Part model, mm, in its own coordinate system. Face numbers are marked on the shaded views. A direction names the side the tool comes from. Coordinates: 2 decimals unless noted, no trailing zeros. Write each loop counter-clockwise with the first axis right and the second up, starting at its lowest first coordinate (ties: lowest second). Pieces come first, ordered by that corner, then holes. Notation, with made-up numbers: (-3.75, 80) - (46.25, 80) arc R27 ccw to (46.25, 112) - close; hole circle Ø2 at (-3, -13.5). An arc over 180 degrees is marked (long way). Write each question's results on one line, items separated by ' | '.
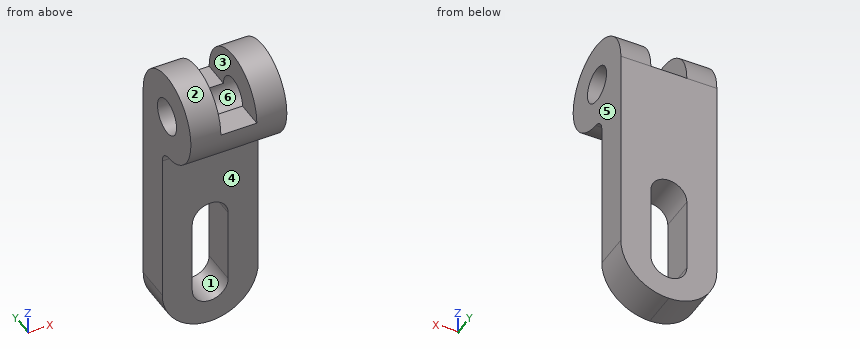
from build123d import *

# Parameters (mm, degrees)
F0_R     = 6
F1_DEPTH = 32
F3_DEPTH = 15.001
F4_W     = 12
F4_H     = 15
F5_DEPTH = 30.001


# Not quite as in the source:
# - a feature names something its author has since deleted; it is built from what else it names


with BuildPart() as f1:
    # F0 (on Right) → F1 (new body)
    with BuildSketch(Plane.YZ):
        with BuildLine():
            Line((15, -86), (15, 0))
            ThreePointArc((15, 0), (-10.3237080242, 10.8821437517), (-0.7894736842, -14.9792099692))
            ThreePointArc((-0.7894736842, -14.9792099692), (1.9019050004, -16.2206771546), (3, -18.973665961))
            Line((3, -18.973665961), (3, -86))
            Line((3, -86), (15, -86))
        make_face()
        Circle(F0_R, mode=Mode.SUBTRACT)
    extrude(amount=-F1_DEPTH)

    # F2 (on Front) → F3 (cut, through all)
    with BuildSketch(Plane.XZ):
        with BuildLine():
            ThreePointArc((-16, -86), (-27.313708499, -81.313708499), (-32, -70))
            Line((-32, -70), (-32, -86))
            Line((-32, -86), (-16, -86))
        make_face()
        with BuildLine():
            ThreePointArc((0, -70), (-4.686291501, -81.313708499), (-16, -86))
            Line((-16, -86), (0, -86))
            Line((0, -86), (0, -70))
        make_face()
        with BuildLine():
            Line((-10, -72.1075447824), (-10, -47.1075447824))
            ThreePointArc((-10, -47.1075447824), (-16, -41.1075447824), (-22, -47.1075447824))
            Line((-22, -47.1075447824), (-22, -72.1075447824))
            ThreePointArc((-22, -72.1075447824), (-16, -78.1075447824), (-10, -72.1075447824))
        make_face()
    extrude(amount=-F3_DEPTH, mode=Mode.SUBTRACT)

    # F4 (on face) → F5 (cut, through all)
    with BuildSketch(Plane(origin=(0, 15, 0), x_dir=(-1, 0, 0), z_dir=(0, 1, 0))):
        with Locations((16, 7.5)):
            Rectangle(F4_W, F4_H)
    extrude(amount=-F5_DEPTH, mode=Mode.SUBTRACT)


solid = f1.part
(1) 3-axis set-ups, long thin cutter, end or side, ignore diameter. For the marked faces 1, 2 and 3: which of +Z, -Z, +X, -X, +Y, -Y reach the whole face in a straight line?
Return value:
face 1: +Y, -Y | face 2: +X, -X | face 3: +Z, +Y, -Y
(2) Two-plate mould, pull along Y, no slides. Class the marked faces 4, 5 and 6: released by +Y, released by -Y, zero draft, split by the parting line, or undercut.
Return value:
face 4: released by -Y | face 5: zero draft | face 6: undercut
(3) Saw through at D-D on y = -4. Write the cut outline in (x, z).
Return value:
outline: (-32, -14.46) - (0, -14.46) - (0, -4.47) - (-32, -4.47) - close; (-32, 4.47) - (-22, 4.47) - (-22, 14.46) - (-32, 14.46) - close; (-10, 4.47) - (0, 4.47) - (0, 14.46) - (-10, 14.46) - close
(4) Saw through at C-C on x = -17. Write the cut outline in (y, z), then the cut area to 3 significant figures.
Return value:
outline: (-15, 0) arc R15 ccw to (-0.79, -14.98) arc R4 cw to (3, -18.97) - (3, -41.19) - (15, -41.19) - (15, 0) - (6, 0) arc R6 cw to (-6, 0) - close; (3, -85.97) - (15, -85.97) - (15, -78.02) - (3, -78.02) - close | area: 758 mm^2
(5) Wall check: line 1 (Y direction, x = -24, z = 0); line 2 (Y direction, x = -7.5, z = -27); line 3 (Y direction, x = -9.5, z = 3.5). Give the ranges that are in metal, low to high. Write a range as from..to.
Return value:
line 1: y = -15..-6, 6..15 | line 2: y = 3..15 | line 3: y = -14.59..-4.87, 4.87..14.59
(6) Saw through at A-A on z = -75.5. Write the cut outline in (x, y).
Return value:
outline: (-31.02, 3) - (-20.95, 3) - (-20.95, 15) - (-31.02, 15) - close; (-11.05, 3) - (-0.98, 3) - (-0.98, 15) - (-11.05, 15) - close
(7) Saw through at B-B on y = 12. Write the cut outline in (x, z), then the cut area to 3 significant figures.
Return value:
outline: (-32, -70) arc R16 ccw to (0, -70) - (0, 9) - (-10, 9) - (-10, 0) - (-22, 0) - (-22, 9) - (-32, 9) - close; hole (-22, -72.11) arc R6 ccw to (-10, -72.11) - (-10, -47.11) arc R6 ccw to (-22, -47.11) - close | area: 2,410 mm^2
(8) Flat gauge pins, fed straight in: P1, Ø10, axis at x = -14, y = -10, coming from the +Z side; P2, Ø12, axis at y = 1.5, z = 10.5, coming from the +X side; P3, Ø2, axis at x = -21, y = 0, coming from the -Z side; P4, Ø5, axis at x = -22, y = 1, coming from the -Z side. Where does each tip first touch, or does it go through?
Return value:
P1: stops at z = 13.27 | P2: stops at x = 0 | P3: stops at z = -15.51 | P4: stops at z = -85.35
